Source: CAD feature listing. Evaluate the final solid. Frame: model axes, mm. Face numbers are marked on the shaded views. A direction names the side the tool comes from. Give positions to 0.01 mm unless a question says otherwise; leave off trailing zeros. Order: outer loops, then holes, each group sorted by start corner. A loop starts at its lowest first (then second) coordinate and runs counter-clockwise, first axis right, second up. Notation, with made-up numbers: M 30.5,74 L 75.5,74 A18 ccw 75.5,83 Z; hole C 56.25,12.25 d7. An arc over 180 degrees is marked long. One line per question, with ' | ' between items. Start each with the question number.
Autodesk Inventor part; units mm, degrees
ref_plane "YZ Plane" through (0, 0, 0) normal (1, 0, 0) x (0, 1, 0)
ref_plane "XZ Plane" through (0, 0, 0) normal (0, 1, 0) x (-1, 0, 0)
ref_plane "XY Plane" through (0, 0, 0) normal (0, 0, 1) x (1, 0, 0)
sketch "Sketch1" plane through (0, 0, 0) normal (0, 0, 1) x (1, 0, 0)
  circle A0 centre (0, 0) radius 15.875
  circle A1 centre (0, 0) radius 2.75
  dimension "d0" = 31.75
  dimension "d1" = 5.5
extrude "Extrusion1" add sketch "Sketch1" along normal blind 6
sketch "Sketch2" plane through (0, 0, 6) normal (0, 0, 1) x (1, 0, 0)
  line L0 (-17.145, 8.763) -> (-8.255, 8.763)
  line L1 (-8.255, 8.763) -> (-8.255, -8.763)
  line L2 (-8.255, -8.763) -> (-17.145, -8.763)
  line L3 (-17.145, -8.763) -> (-17.145, 8.763)
  line L4 (8.89, 5.08) -> (16.51, 5.08)
  line L5 (16.51, 5.08) -> (16.51, -5.08)
  line L6 (16.51, -5.08) -> (8.89, -5.08)
  line L7 (8.89, -5.08) -> (8.89, 5.08)
  line L8 (-12.7, 8.763) -> (-12.7, -8.763) construction
  line L9 (12.7, 5.08) -> (12.7, -5.08) construction
  point P0 (0, 0)
  point P1 (-8.255, 0)
  point P2 (8.89, 0)
  dimension "d4" = 8.89
  dimension "d5" = 7.62
  dimension "d6" = 10.16
  dimension "d7" = 12.7
  dimension "d8" = 12.7
  dimension "d9" = 17.526
extrude "Extrusion2" cut sketch "Sketch2" against normal through all
sketch "Sketch3" plane through (0, 0, 6) normal (0, 0, 1) x (1, 0, 0)
  line L0 (-21.6805, 12.7) -> (-8.255, 12.7)
  line L1 (-8.255, 12.7) -> (-8.255, -12.7)
  line L2 (-8.255, -12.7) -> (-21.6805, -12.7)
  line L3 (-21.6805, -12.7) -> (-21.6805, 12.7)
  line L4 (-8.255, 8.763) -> (-8.255, -8.763)
  line L5 (8.89, 12.7) -> (29.1291, 12.7)
  line L6 (29.1291, 12.7) -> (29.1291, -12.7)
  line L7 (29.1291, -12.7) -> (8.89, -12.7)
  line L8 (8.89, -12.7) -> (8.89, 12.7)
  line L9 (8.89, -5.08) -> (8.89, 5.08)
  point P0 (0, 0)
  point P1 (-21.6805, 0)
  dimension "d12" = 25.4
extrude "Extrusion3" cut sketch "Sketch3" against normal blind 4
properties part number "fakebattergasket3"
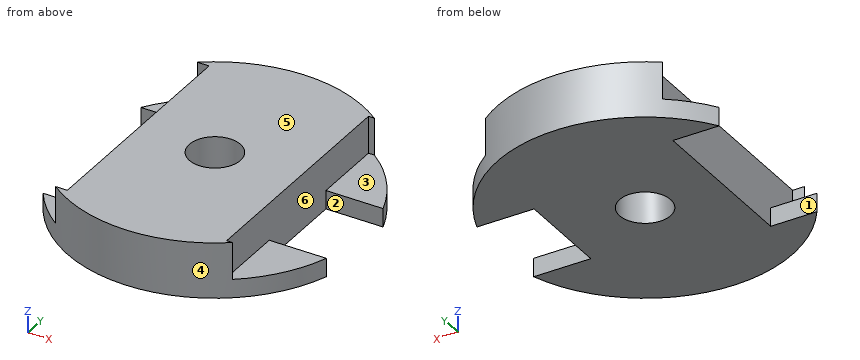
Item 1: Cut plane A-A on y = 0. Return the cut outline in (x, z) (3 decimals), and give its area (3 significant figures).
Item 2: Mould query, pull axis Y, two halves, no side actions, for the marked faces 4, 5 and 6. Classes: pulls with the +Y half, pulls with the -Y half, needs draft (parallel to the pull), parting line crosses it, or undercut.
Item 3: Reachability of the marked faces 1, 2 and 3 from +Z, -Z, +X, -X, +Y, -Y: full face, straight path, thin tool, end or side. Return the list, or none.
Item 4: Cut plane C-C on z = 3.55. Return the cut outline in (x, y) (3 decimals), and give its area (3 significant figures).
Item 5: Pin query (flat end, axial travel): pin 1 Ø1 at (x, z) = (12, 1.5) entering from +Y; pin 2 Ø0.6 at (x, z) = (-11, 1.5) entering from +Y; pin 3 Ø0.6 at (x, z) = (11.5, 0.5) entering from -Y. Return the tip coordinate at first contact, or that it passes through.
Item 6: Cut plane B-B on x = 0. Return the cut outline in (y, z) (3 decimals), and give its area (4 significant figures).
Item 7: Line query: line 1 (Y direction, x = 0, z = 2.75) (3 decimals); line 2 (X direction, y = -6.5, z = 2.6) (3 decimals); line 3 (Z direction, x = 11.5, y = -10.5). Output: solid intervals per line, ascending.
Item 8: Cut plane D-D on y = -11. Return the cut outline in (x, z) (3 decimals).
Results are:
1) outline: M -8.255,0 L -2.75,0 L -2.75,6 L -8.255,6 Z; M 2.75,0 L 8.89,0 L 8.89,6 L 2.75,6 Z | area: 69.9 mm2
2) face 4: pulls with the -Y half | face 5: needs draft | face 6: undercut
3) face 1: +Z, -Z, -X | face 2: +Z, -Z, +X | face 3: +Z, +X
4) outline: M -9.525,-12.7 A15.875 ccw 9.525,-12.7 L 8.89,-12.7 L 8.89,12.7 L 9.525,12.7 A15.875 ccw -9.525,12.7 L -8.255,12.7 L -8.255,-12.7 Z; hole C 0,0 d5.5 | area: 494 mm2
5) pin 1: stops at y = 10.94 | pin 2: stops at y = 11.73 | pin 3: stops at y = -11.25
6) outline: M -15.875,0 L -2.75,0 L -2.75,6 L -15.875,6 Z; M 2.75,0 L 15.875,0 L 15.875,6 L 2.75,6 Z | area: 157.5 mm2
7) line 1: y = -15.875 to -2.75, 2.75 to 15.875 | line 2: x = -8.255 to 8.89 | line 3: z = 0 to 2
8) outline: M -11.446,0 L 11.446,0 L 11.446,2 L 8.89,2 L 8.89,6 L -8.255,6 L -8.255,2 L -11.446,2 Z
